from build123d import *

# Parameters (mm, degrees)
F1_DEPTH = 24
F2_R     = 1.7
F3_DEPTH = 25


with BuildPart() as f1:
    # F0 (on Front) → F1 (new body)
    with BuildSketch(Plane.XZ):
        with BuildLine():
            ThreePointArc((-7.7, -0.172106), (0, 7.527894), (7.7, -0.172106))
            Line((7.7, -0.172106), (15.699692, -0.270456))
            Line((15.699692, -0.270456), (27.699692, -0.270456))
            Line((27.699692, -0.270456), (27.699692, 6.073763))
            Line((27.699692, 6.073763), (14.404135, 6.073763))
            ThreePointArc((14.404135, 6.073763), (0, 15.527894), (-14.404135, 6.073763))
            Line((-14.404135, 6.073763), (-27.698785, 6.073763))
            Line((-27.698785, 6.073763), (-27.698785, 0.073763))
            Line((-27.698785, 0.073763), (-15.699692, -0.073756))
            Line((-15.699692, -0.073756), (-7.7, -0.172106))
        make_face()
    extrude(amount=F1_DEPTH)

    # F2 (on face) → F3 (cut)
    with BuildSketch(Plane(origin=(-0.003279, 0, -0.266731), x_dir=(0.999924, 0, -0.012293), z_dir=(-0.012293, 0, -0.999924))):
        with Locations((-21.7, 12)):
            Circle(F2_R)
        with Locations((21.7, 12)):
            Circle(F2_R)
    extrude(amount=-F3_DEPTH, mode=Mode.SUBTRACT)


solid = f1.part
Input: part model. Units: mm. Frame: model coordinates. A direction names the side the tool comes from. Round coordinates to 2 decimals unless told otherwise and drop trailing zeros. Loops run counter-clockwise (first coordinate to the right, second up) from the corner with the lowest first, then second, coordinate; pieces in that order, holes last. Notation, with made-up numbers: (61, 45.25) -> (113, 45.25) arc R30 cw to (113, 78.25) -> close; hole circle Ø2 at (7, 26.25). An arc over 180 degrees is marked (long way). Answer as a JSON object with one key per item and string values. Group by question number.
1) Ray query, L1, parallel to X at y = -11.5, z = 2.75; L2, parallel to Z at x = 17.5, y = -13.5; L3, parallel to X at y = -19.25, z = 3. Return the intervals inside material, ascending.
2) Section query A-A on y = -1.75. Output: boundary loops of the cut face in (x, z), plus the area to 3 significant figures.
3) Draft query along Y for faces 4 (the cylindrical face through (20.04, -12.07, 2.88)), 5 (the flat face through (0, 0, 8)), 6 (the cylindrical face through (-0.169, -11.832, 7.526)), 7 (the cylindrical face through (-20.094, -11.349, 2.985)). Return one class per face: +Y half, -Y half, draft (parallel to the pull), parting line (faces both ways), or undercut.
4) Section query B-B on z = 7. Output: boundary loops of the cut face in (x, y).
5) Reachability of faces 1 (the flat face through (19.7, -11.8, 6.074)), 2 (the flat face through (-19, -12, 6.074)), 3 (the cylindrical face through (0.255, -11.832, 15.526)) from +Z, -Z, +X, -X, +Y, -Y: full face, straight path, thin tool, end or side. Return the list, or none.
6) Pin query (flat end, axial travel): pin 1 (4 mm diameter, centred on x = 23.5, y = -9.5, fed in from +Z); pin 2 (2 mm diameter, centred on x = 12.5, y = -12, fed in from +Z); pin 3 (12 mm diameter, centred on x = -20, y = -6, fed in from -Z). Return the tip coordinate at first contact, or that it passes through.
7) Section query D-D on x = 0. Output: boundary loops of the cut face in (y, z).
8) Section query C-C on z = 1.25. State how many separate pieces and enclosed holes the cut face has, plus the area to 3 significant figures.
Reply:
{
 "1": {"L1": "x = -27.7 to -23.29, -20.04 to -7.12, 7.12 to 20.11, 23.36 to 27.7", "L2": "z = -0.27 to 6.07", "L3": "x = -27.7 to -7.02, 7.02 to 27.7"},
 "2": {"outline": "(-27.7, 0.07) -> (-7.7, -0.17) arc R7.7 cw to (7.7, -0.17) -> (15.7, -0.27) -> (27.7, -0.27) -> (27.7, 6.07) -> (14.4, 6.07) arc R15.7 ccw to (-14.4, 6.07) -> (-27.7, 6.07) -> close", "area": "448 mm2"},
 "3": {"face 4": "undercut", "face 5": "+Y half", "face 6": "draft", "face 7": "undercut"},
 "4": {"outline": "(-13.97, -24) -> (-2.8, -24) -> (-2.8, 0) -> (-13.97, 0) -> close; (2.8, -24) -> (13.97, -24) -> (13.97, 0) -> (2.8, 0) -> close"},
 "5": {"face 1": "+Z, +X, +Y, -Y", "face 2": "+Z, -X, +Y, -Y", "face 3": "+Z, +Y, -Y"},
 "6": {"pin 1": "stops at z = 6.07", "pin 2": "stops at z = 10.52", "pin 3": "stops at z = -0.09"},
 "7": {"outline": "(-24, 7.53) -> (0, 7.53) -> (0, 15.53) -> (-24, 15.53) -> close"},
 "8": {"separate pieces": "2", "enclosed holes": "2", "area": "948 mm2"}
}
